Verification items for the finished model (mm, model axes). A direction names the side the tool comes from. Round coordinates to 2 decimals unless told otherwise and drop trailing zeros. Write each loop counter-clockwise with the first axis right and the second up, starting at its lowest first coordinate (ties: lowest second). Pieces come first, ordered by that corner, then holes. Notation, with made-up numbers: (41, -16.5) -> (87, -16.5) arc R30 cw to (87, 13.5) -> close; hole circle Ø5 at (62.5, 83.5). An arc over 180 degrees is marked (long way). Answer as a JSON object with one key per item and string values. Group by question number.
(1) Sectioned sample at B-B on x = 1. Record the cut outline in (y, z).
(2) Draft check along X on faces 1 (the face through (-15, 6, 0)), 2 (the face through (-10.9, 2, -4)). Enter one of: released by +X, released by -X, zero draft, split by the parting line, or undercut.
(3) Sectioned sample at D-D on x = -4.75. Record the cut outline in (y, z), and give its area (3 significant figures).
(4) Gauge pin test, flat end, axial feed: pin 1 Ø12 at (x, z) = (6, 6.5) entering from +Y. Record the tip position at first contact, or that the pin passes through.
(5) Sectioned sample at A-A on z = -14. Record the cut outline in (x, y).
(6) Sectioned sample at C-C on y = 7. Record the cut outline in (x, z).
(7) Scan lines: L1, parallel to X at y = 1, z = 6.5; L2, parallel to X at y = 2.25, z = 17; L3, parallel to X at y = 5.25, z = -6.5. Record each from-to range of solid material in increasing order. Write a range as from..to.
(8) Set-up check for faces 3 (the face through (10.9, 2, -4)), 4 (the face through (-13, 8, 2)): record each of +Z, -Z, +X, -X, +Y, -Y from which the full face is reachable in a straight line by a thin tool's end or side.
```python
from build123d import *

# Parameters (mm, degrees)
SKETCH1_W           = 30
SKETCH1_H           = 60
BOSS_EXTRUDE1_DEPTH = 3
SKETCH2_W           = 12.8
SKETCH2_H           = 6
SKETCH2_W_2         = 7.8
CUT_EXTRUDE1_DEPTH  = 3
SKETCH4_W           = 30
SKETCH4_H           = 60
SKETCH4_W_2         = 26
SKETCH4_H_2         = 56
BOSS_EXTRUDE2_DEPTH = 10
SKETCH5_W           = 26
SKETCH5_H           = 8
SKETCH5_H_2         = 5
BOSS_EXTRUDE3_DEPTH = 10
FILLET1_R           = 2


with BuildPart() as part:
    # Sketch1 → Boss-Extrude1 (new body)
    with BuildSketch(Plane(origin=(0, 0, 0), x_dir=(1, 0, 0), z_dir=(0, 1, 0))):
        Rectangle(SKETCH1_W, SKETCH1_H)
    extrude(amount=BOSS_EXTRUDE1_DEPTH)

    # Sketch2 → Cut-Extrude1 (cut)
    with BuildSketch(Plane(origin=(0, 3, 0), x_dir=(1, 0, 0), z_dir=(0, 1, 0))):
        with Locations((0, -19)):
            Rectangle(SKETCH2_W, SKETCH2_H)
        with Locations((-7, 4)):
            Rectangle(SKETCH2_W_2, SKETCH2_H)
        with Locations((-7, -8)):
            Rectangle(SKETCH2_W_2, SKETCH2_H)
        with Locations((-7, 16)):
            Rectangle(SKETCH2_W_2, SKETCH2_H)
        with Locations((7, -8)):
            Rectangle(SKETCH2_W_2, SKETCH2_H)
        with Locations((7, 4)):
            Rectangle(SKETCH2_W_2, SKETCH2_H)
        with Locations((7, 16)):
            Rectangle(SKETCH2_W_2, SKETCH2_H)
    extrude(amount=-CUT_EXTRUDE1_DEPTH, mode=Mode.SUBTRACT)

    # Sketch4 → Boss-Extrude2 (add)
    with BuildSketch(Plane(origin=(0, 3, 0), x_dir=(1, 0, 0), z_dir=(0, 1, 0))):
        Rectangle(SKETCH4_W, SKETCH4_H)
        Rectangle(SKETCH4_W_2, SKETCH4_H_2, mode=Mode.SUBTRACT)
    extrude(amount=BOSS_EXTRUDE2_DEPTH)

    # Sketch5 → Boss-Extrude3 (add)
    with BuildSketch(Plane(origin=(0, 3, 0), x_dir=(1, 0, 0), z_dir=(0, 1, 0))):
        with Locations((0, 24)):
            Rectangle(SKETCH5_W, SKETCH5_H)
        with Locations((0, -25.5)):
            Rectangle(SKETCH5_W, SKETCH5_H_2)
    extrude(amount=BOSS_EXTRUDE3_DEPTH)

    # Fillet1
    fillet1_edges = [part.edges().sort_by_distance(p)[0] for p in [
        (15, 6.5, 30),
        (-15, 6.5, 30),
        (-15, 6.5, -30),
        (15, 6.5, -30),
    ]]
    fillet(fillet1_edges, radius=FILLET1_R)


solid = part.part
```
Computed values:
{
 "1": {"outline": "(0, -30) -> (13, -30) -> (13, -20) -> (3, -20) -> (3, 16) -> (0, 16) -> close; (0, 22) -> (3, 22) -> (3, 23) -> (13, 23) -> (13, 30) -> (0, 30) -> close"},
 "2": {"face 1": "released by -X", "face 2": "undercut"},
 "3": {"outline": "(0, -30) -> (13, -30) -> (13, -20) -> (3, -20) -> (3, -19) -> (0, -19) -> close; (0, -13) -> (3, -13) -> (3, -7) -> (0, -7) -> close; (0, -1) -> (3, -1) -> (3, 5) -> (0, 5) -> close; (0, 11) -> (3, 11) -> (3, 16) -> (0, 16) -> close; (0, 22) -> (3, 22) -> (3, 23) -> (13, 23) -> (13, 30) -> (0, 30) -> close", "area": "278 mm2"},
 "4": {"pin 1": "y = 3"},
 "5": {"outline": "(-15, 0) -> (-10.9, 0) -> (-10.9, 3) -> (-13, 3) -> (-13, 13) -> (-15, 13) -> close; (-3.1, 0) -> (3.1, 0) -> (3.1, 3) -> (-3.1, 3) -> close; (10.9, 0) -> (15, 0) -> (15, 13) -> (13, 13) -> (13, 3) -> (10.9, 3) -> close"},
 "6": {"outline": "(-15, -28) arc R2 ccw to (-13, -30) -> (13, -30) arc R2 ccw to (15, -28) -> (15, 28) arc R2 ccw to (13, 30) -> (-13, 30) arc R2 ccw to (-15, 28) -> close; hole (-13, -20) -> (13, -20) -> (13, 23) -> (-13, 23) -> close"},
 "7": {"L1": "-15..-10.9, -3.1..3.1, 10.9..15", "L2": "-15..-6.4, 6.4..15", "L3": "-15..-13, 13..15"},
 "8": {"face 3": "+Y, -Y", "face 4": "+Y"}
}
